from build123d import *

# Parameters (mm, degrees)
SKETCH2_W             = 10
SKETCH2_H             = 101.6
BOSS_EXTRUDE1_DEPTH   = 139.7
BOSS_EXTRUDE1_2_DEPTH = 139.7
SKETCH2_3_W           = 10
SKETCH2_3_H           = 101.6
SKETCH2_3_W_2         = 80
BOSS_EXTRUDE2_DEPTH   = 5
SKETCH3_R             = 14.605
CUT_EXTRUDE1_DEPTH    = 117
SKETCH4_W             = 16.851782798
SKETCH4_H             = 139.7
CUT_EXTRUDE2_DEPTH    = 119
FILLET14_R            = 15
FILLET2_R             = 10
SKETCH7_R             = 1.6
CUT_EXTRUDE4_DEPTH    = 21
BOSS_EXTRUDE3_START   = 80
SKETCH8_R             = 14.75414129
SKETCH8_R_2           = 7.62
BOSS_EXTRUDE3_DEPTH   = 3
SKETCH9_R             = 1.905
CUT_EXTRUDE5_DEPTH    = 145.7
CUT_EXTRUDE6_DEPTH    = 10
FILLET4_R             = 25
SKETCH10_R            = 2.4003
CUT_EXTRUDE7_DEPTH    = 10
SKETCH11_R            = 4.7
CUT_EXTRUDE9_DEPTH    = 10
CHAMFER1_SIZE         = 1.778
SKETCH12_R            = 2.921
CUT_EXTRUDE10_DEPTH   = 3.302


with BuildPart() as part:
    # Sketch2 → Boss-Extrude1 (new body)
    with BuildSketch(Plane(origin=(0, 0, 0), x_dir=(1, 0, 0), z_dir=(0, 1, 0))):
        with Locations((-45, 0)):
            Rectangle(SKETCH2_W, SKETCH2_H)
    extrude(amount=BOSS_EXTRUDE1_DEPTH)



with BuildPart() as body_2:
    # Sketch2 → Boss-Extrude1 2 (new body)
    with BuildSketch(Plane(origin=(0, 0, 0), x_dir=(1, 0, 0), z_dir=(0, 1, 0))):
        with Locations((45, 0)):
            Rectangle(SKETCH2_W, SKETCH2_H)
    extrude(amount=BOSS_EXTRUDE1_2_DEPTH)


with BuildPart() as part_1:
    add(part.part)

    add(body_2.part)  # Boss-Extrude2 merges body 2
    # Sketch2<3> → Boss-Extrude2 (add)
    with BuildSketch(Plane(origin=(0, 0, 0), x_dir=(1, 0, 0), z_dir=(0, 1, 0))):
        with Locations((45, 0)):
            Rectangle(SKETCH2_3_W, SKETCH2_3_H)
        Rectangle(SKETCH2_3_W_2, SKETCH2_3_H)
        with Locations((-45, 0)):
            Rectangle(SKETCH2_3_W, SKETCH2_3_H)
    extrude(amount=-BOSS_EXTRUDE2_DEPTH)

    # Sketch3 → Cut-Extrude1 (cut)
    with BuildSketch(Plane.ZY.offset(50)):
        with Locations((0, 109.7)):
            Circle(SKETCH3_R)
    extrude(amount=-CUT_EXTRUDE1_DEPTH, mode=Mode.SUBTRACT)

    # Sketch4 → Cut-Extrude2 (cut)
    with BuildSketch(Plane(origin=(50, 0, 0), x_dir=(0, 0, -1), z_dir=(1, 0, 0))):
        with Locations((-42.374108601, 69.85)):
            Rectangle(SKETCH4_W, SKETCH4_H)
        with Locations((42.374108601, 69.85)):
            Rectangle(SKETCH4_W, SKETCH4_H)
    extrude(amount=-CUT_EXTRUDE2_DEPTH, mode=Mode.SUBTRACT)

    # Fillet14
    fillet14_edges = [part_1.edges().sort_by_distance(p)[0] for p in [
        (45, 139.7, -33.948217202),
        (45, 139.7, 33.948217202),
        (40, 0, 0),
        (-40, 0, 0),
        (-45, 0, 33.948217202),
        (45, 0, 33.948217202),
        (-45, 0, -33.948217202),
        (45, 0, -33.948217202),
    ]]
    fillet(fillet14_edges, radius=FILLET14_R)

    # Fillet2
    fillet2_edges = [part_1.edges().sort_by_distance(p)[0] for p in [
        (50, -2.5, -50.8),
        (-50, -2.5, -50.8),
        (50, -2.5, 50.8),
        (-50, -2.5, 50.8),
    ]]
    fillet(fillet2_edges, radius=FILLET2_R)

    # Sketch7 → Cut-Extrude4 (cut)
    with BuildSketch(Plane(origin=(50, 0, 0), x_dir=(0, 0, -1), z_dir=(1, 0, 0))):
        with Locations((-15.5, 125.2)):
            Circle(SKETCH7_R)
        with Locations((15.5, 125.2)):
            Circle(SKETCH7_R)
        with Locations((15.5, 94.2)):
            Circle(SKETCH7_R)
        with Locations((-15.5, 94.2)):
            Circle(SKETCH7_R)
    extrude(amount=-CUT_EXTRUDE4_DEPTH, mode=Mode.SUBTRACT)

    # Sketch8 → Boss-Extrude3 (add)
    with BuildSketch(Plane.ZY.offset(-40).offset(BOSS_EXTRUDE3_START)):
        with Locations((0, 109.7)):
            Circle(SKETCH8_R)
        with Locations((0, 109.7)):
            Circle(SKETCH8_R_2, mode=Mode.SUBTRACT)
    extrude(amount=BOSS_EXTRUDE3_DEPTH)

    # Sketch9 → Cut-Extrude5 (cut, through all)
    with BuildSketch(Plane.XZ.offset(5)):
        with Locations((-40.66, 40.66)):
            Circle(SKETCH9_R)
        with Locations((40.66, 40.66)):
            Circle(SKETCH9_R)
        with Locations((-40.66, -40.66)):
            Circle(SKETCH9_R)
        with Locations((40.66, -40.66)):
            Circle(SKETCH9_R)
    extrude(amount=-CUT_EXTRUDE5_DEPTH, mode=Mode.SUBTRACT)

    # Sketch5 → Cut-Extrude6 (cut)
    with BuildSketch(Plane(origin=(0, 0, 0), x_dir=(1, 0, 0), z_dir=(0, 1, 0))):
        with BuildLine():
            Line((-1.917657947, 2.032), (1.917657947, 2.032))
            ThreePointArc((1.917657947, 2.032), (0, -2.794), (-1.917657947, 2.032))
        make_face()
    extrude(amount=-CUT_EXTRUDE6_DEPTH, mode=Mode.SUBTRACT)

    # Fillet4
    fillet4_edges = [part_1.edges().sort_by_distance(p)[0] for p in [
        (-45, 139.7, 33.948217202),
        (-45, 139.7, -33.948217202),
    ]]
    fillet(fillet4_edges, radius=FILLET4_R)

    # Sketch10 → Cut-Extrude7 (cut)
    with BuildSketch(Plane(origin=(0, 0, 0), x_dir=(1, 0, 0), z_dir=(0, 1, 0))):
        with Locations((-5.856308805, 5.856308805)):
            Circle(SKETCH10_R)
        with Locations((5.856308805, 5.856308805)):
            Circle(SKETCH10_R)
        with Locations((-5.856308805, -5.856308805)):
            Circle(SKETCH10_R)
        with Locations((5.856308805, -5.856308805)):
            Circle(SKETCH10_R)
    extrude(amount=-CUT_EXTRUDE7_DEPTH, mode=Mode.SUBTRACT)

    # Sketch11 → Cut-Extrude9 (cut)
    with BuildSketch(Plane(origin=(0, 0, 0), x_dir=(1, 0, 0), z_dir=(0, 1, 0))):
        with Locations((-40.66, -40.66)):
            Circle(SKETCH11_R)
        with Locations((40.66, -40.66)):
            Circle(SKETCH11_R)
        with Locations((-40.66, 40.66)):
            Circle(SKETCH11_R)
        with Locations((40.66, 40.66)):
            Circle(SKETCH11_R)
    extrude(amount=CUT_EXTRUDE9_DEPTH, mode=Mode.SUBTRACT)

    # Chamfer1
    chamfer1_edges = [part_1.edges().sort_by_distance(p)[0] for p in [
        (38.755, -5, 40.66),
        (-42.565, -5, -40.66),
        (38.755, -5, -40.66),
        (-42.565, -5, 40.66),
    ]]
    chamfer(chamfer1_edges, length=CHAMFER1_SIZE)

    # Sketch12 → Cut-Extrude10 (cut)
    with BuildSketch(Plane.ZY.offset(-40)):
        with Locations((-15.5, 125.2)):
            Circle(SKETCH12_R)
        with Locations((15.5, 125.2)):
            Circle(SKETCH12_R)
        with Locations((-15.5, 94.2)):
            Circle(SKETCH12_R)
        with Locations((15.5, 94.2)):
            Circle(SKETCH12_R)
    extrude(amount=-CUT_EXTRUDE10_DEPTH, mode=Mode.SUBTRACT)


solid = part_1.part
Read the model definition and answer for the solid it produces. Units are mm, in the model's axes. A direction names the side the tool comes from. Give positions to 0.01 mm unless a question says otherwise; leave off trailing zeros. Write each loop counter-clockwise with the first axis right and the second up, starting at its lowest first coordinate (ties: lowest second). Pieces come first, ordered by that corner, then holes. Notation, with made-up numbers: (89.5, -1.5) - (114.5, -1.5) arc R24 ccw to (114.5, 30.5) - close; hole circle Ø7 at (-4, -34.5). An arc over 180 degrees is marked (long way). Use CSV: the item, a comma, the result in double quotes. Start each with the question number.
(1) Find section B-B (y = 109.7). Give the vertices of the cut face in (x, z) (3 decimals), plus the area to 3 significant figures.
(2) Find section C-C (y = 26.5). Give the vertices of the cut face in (x, z), plus the area to 3 significant figures.
(3) Find section D-D (z = 24). Give the vertices of the cut face in (x, y).
(4) Find section A-A (x = 0). Give the vertices of the cut face in (y, z), plus the area to 3 significant figures.
(5) For faces 1 (the cylindrical face through (46.698, 95.786, 15.708)), 2 (the flat face through (43, 0, 41)), 3 (the cylindrical face through (-46.549, 122.015, 7.852)), 4 (the flat face through (43.302, 93, 17)), determine the directions among +Z, -Z, +X, -X, +Y, -Y from which every point of the face is accessible in a straight line to the end or side of a thin tool.
(6) Given P1, Ø1.9, axis at y = 94.2, z = 15.5, coming from the +X side; P2, Ø8, axis at x = -43, y = 72, coming from the +Z side; P3, Ø5, axis at x = -40.66, z = 40.66, coming from the -Y side; P4, Ø8.5, axis at x = -40.66, z = -40.66, coming from the -Y side, each flat-ended and moving along its own axis, determine where each tip first touches the part or whether it passes through.
(7) Consider line 1 along X through (y, z) = (38, 2.5); line 2 along X through (y, z) = (-1, -40); line 3 along Y through (x, z) = (42, 15). Determine where each line is inside the solid, lowest interval first.
(8) Determine the mould class of faces 5 (the cylindrical face through (-45.1, 132.2, 26.8)), 6 (the cylindrical face through (-4.749, -2.465, 7.986)), 7 (the flat face through (43.302, 124, -14)), 8 (the flat face through (-50, 52, 1)) for opening direction X: +X half, -X half, draft (parallel to the pull), parting line (faces both ways), or undercut.
Findings below:
1,outline,"(-50, -33.948) - (-40, -33.948) - (-40, -7.62) - (-43, -7.62) - (-43, -14.605) - (-50, -14.605) - close; (-50, 14.605) - (-43, 14.605) - (-43, 7.62) - (-40, 7.62) - (-40, 33.948) - (-50, 33.948) - close; (40, -33.948) - (50, -33.948) - (50, -14.605) - (40, -14.605) - close; (40, 14.605) - (50, 14.605) - (50, 33.948) - (40, 33.948) - close"
1,area,"816 mm2"
2,outline,"(-50, -33.95) - (-40, -33.95) - (-40, 33.95) - (-50, 33.95) - close; (40, -33.95) - (50, -33.95) - (50, 33.95) - (40, 33.95) - close"
2,area,"1,360 mm2"
3,outline,"(-50, -5) - (50, -5) - (50, 138.82) - (40, 138.82) - (40, 15) arc R15 cw to (25, 0) - (-25, 0) arc R15 cw to (-40, 15) - (-40, 134.66) - (-50, 134.66) - close"
4,outline,"(-5, -50.8) - (0, -50.8) - (0, -2.03) - (-5, -2.03) - close; (-5, 2.79) - (0, 2.79) - (0, 50.8) - (-5, 50.8) - close"
4,area,"484 mm2"
5,face 1,"+X"
5,face 2,"+Y"
5,face 3,"-X"
5,face 4,"none"
6,P1,"x = -40"
6,P2,"z = 33.95"
6,P3,"y = -3.82"
6,P4,"y = -5"
7,line 1,"-50 to -40, 40 to 50"
7,line 2,"-50 to -42.45, -38.87 to 38.87, 42.45 to 50"
7,line 3,"-5 to 91.32, 97.08 to 122.32, 128.08 to 139.7"
8,face 5,"draft"
8,face 6,"undercut"
8,face 7,"undercut"
8,face 8,"-X half"
